Here's how the part is built. I have some questions about the finished solid (model axes, mm). Face numbers are marked on the shaded views. Round coordinates to 2 decimals unless told otherwise and drop trailing zeros. Write each loop counter-clockwise with the first axis right and the second up, starting at its lowest first coordinate (ties: lowest second). Pieces come first, ordered by that corner, then holes. Notation, with made-up numbers: (-39.5, -15) - (17.5, -15) arc R20 ccw to (17.5, 10) - close; hole circle Ø6 at (-36.75, 17.25). An arc over 180 degrees is marked (long way). Use one line per item in the form item = value. Start each with the question number.
1. I want a section at A-A, the plane x = -0.25. List the corners of the cut face in (y, z) for me.
2. I want a section at D-D, the plane z = 9. List the corners of the cut face in (x, y) for me (1 decimal), plus the area to 3 significant figures.
3. We'd pull the mould along Y, two halves only. Please class the marked faces 1, 2 and 3: +Y half, -Y half, draft (parallel to the pull), parting line (faces both ways), or undercut.
4. If I drill on line 1 along Y through (x, z) = (0, 7.75); line 2 along Y through (x, z) = (1.75, 13.25); line 3 along X through (y, z) = (8.5, 8), over which ranges is the centre line in solid material (lowest first)?
5. I want a section at B-B, the plane x = -3. List the corners of the cut face in (y, z) for me.
6. Will these pins go through, and if not, where does the flat tip stop? pin 1 (1 mm diameter, centred on x = -3, z = 20.5, fed in from -Y); pin 2 (2 mm diameter, centred on x = 4, z = 4.5, fed in from -Y); pin 3 (4 mm diameter, centred on y = 5.5, z = 3.5, fed in from -X); pin 4 (3.5 mm diameter, centred on x = 0, y = 16.59, fed in from -Z).
7. I want a section at C-C, the plane y = -1.5. List the corners of the cut face in (x, z) for me, plus the area to 3 significant figures.
```python
from build123d import *

# Parameters (mm, degrees)
SKETCH1_R           = 2.286
BOSS_EXTRUDE1_DEPTH = 25.4
SKETCH2_R           = 14.2875
CUT_EXTRUDE1_DEPTH  = 34.583444905
FILLET1_R           = 4.7625


with BuildPart() as part:
    # Sketch1 → Boss-Extrude1 (new body)
    with BuildSketch(Plane.XY):
        with BuildLine():
            Line((4.7625, 16.5862), (4.7625, 0))
            ThreePointArc((4.7625, 0), (0, -4.7625), (-4.7625, 0))
            Line((-4.7625, 0), (-4.7625, 16.5862))
            Line((-4.7625, 16.5862), (-4.7625, 21.447758984))
            Line((-4.7625, 21.447758984), (4.7625, 21.447758984))
            Line((4.7625, 21.447758984), (4.7625, 16.5862))
        make_face()
        Circle(SKETCH1_R, mode=Mode.SUBTRACT)
        with Locations((0, 16.5862)):
            Circle(SKETCH1_R, mode=Mode.SUBTRACT)
    extrude(amount=BOSS_EXTRUDE1_DEPTH)

    # Sketch2 → Cut-Extrude1 (cut, through all)
    with BuildSketch(Plane.XY.offset(25.4)):
        with Locations((-16.67002, 8.2931)):
            Circle(SKETCH2_R)
    extrude(amount=-CUT_EXTRUDE1_DEPTH, mode=Mode.SUBTRACT)

    # Fillet1
    # the kernel refuses this fillet: 4.7625 mm, written as the material it takes off along each edge
    with BuildSketch(Plane(origin=(-4.7625, 0.397302149, -2.281929285), x_dir=(0.5257327344691161, 0.8506498056824712, 0), z_dir=(0, 0, 1))) as fillet1_piece_1:
        with BuildLine():
            CenterArc((1.064900333, -4.760069656), FILLET1_R, 91.830511452, 15.300937173)
            Line((-0.337964996, -0.208874745), (-0.366022303, -0.117850847))
            ThreePointArc((-0.366022303, -0.117850847), (-0.219058541, -0.023412979), (-0.050076043, 0.081024394))
            Line((-0.050076043, 0.081024394), (0.003042572, 0.095201393))
            ThreePointArc((0.003042572, 0.095201393), (0.456385857, 0.087958969), (0.909729142, 0.095201393))
            Line((0.909729142, 0.095201393), (0.912771714, 0))
        make_face()
    extrude(amount=29.963858571, mode=Mode.SUBTRACT)
    with BuildSketch(Plane(origin=(-4.7625, 16.188897851, -3.311119953), x_dir=(0, 1, 0), z_dir=(0, 0, 1))) as fillet1_piece_2:
        with BuildLine():
            CenterArc((1.324447981, -4.7625), FILLET1_R, 90, 28.947133413)
            Line((-0.980613477, -0.594995), (-1.026714706, -0.5116449))
            ThreePointArc((-1.026714706, -0.5116449), (-0.533743292, -0.225909554), (-0.052638652, 0.079383467))
            Line((-0.052638652, 0.079383467), (0, 0.09525))
            Line((0, 0.09525), (1.324447981, 0.09525))
            Line((1.324447981, 0.09525), (1.324447981, 0))
        make_face()
    extrude(amount=32.022239906, mode=Mode.SUBTRACT)


solid = part.part
```
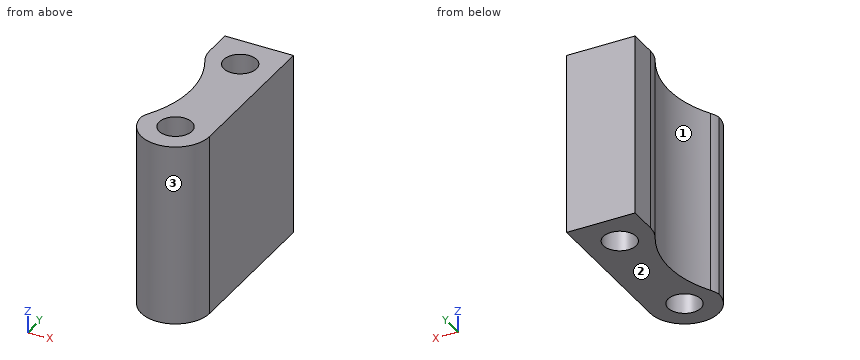
Model answer:
q1.outline = (-4.76, 0) - (-2.27, 0) - (-2.27, 25.4) - (-4.76, 25.4) - close; (2.27, 0) - (14.31, 0) - (14.31, 25.4) - (2.27, 25.4) - close; (18.86, 0) - (21.45, 0) - (21.45, 25.4) - (18.86, 25.4) - close
q2.outline = (-4.8, 0) arc R4.8 ccw to (4.8, 0) - (4.8, 21.4) - (-4.8, 21.4) - (-4.8, 17.5) arc R4.8 ccw to (-4.2, 15.2) arc R14.3 cw to (-4.3, 1.2) arc R4.8 ccw to start; hole circle Ø4.6 at (0, 0); hole circle Ø4.6 at (0, 16.6)
q2.area = 181 mm2
q3.face_1 = undercut
q3.face_2 = draft
q3.face_3 = -Y half
q4.line_1 = -4.76 to -2.29, 2.29 to 14.3, 18.87 to 21.45
q4.line_2 = -4.43 to -1.47, 1.47 to 15.12, 18.06 to 21.45
q4.line_3 = -2.38 to 4.76
q5.outline = (-3.7, 0) - (4.14, 0) - (4.14, 25.4) - (-3.7, 25.4) - close; (12.45, 0) - (21.45, 0) - (21.45, 25.4) - (12.45, 25.4) - close
q6.pin_1 = -4.05
q6.pin_2 = -3.7
q6.pin_3 = -3.21
q6.pin_4 = through
q7.outline = (-4.52, 0) - (-1.73, 0) - (-1.73, 25.4) - (-4.52, 25.4) - close; (1.73, 0) - (4.52, 0) - (4.52, 25.4) - (1.73, 25.4) - close
q7.area = 142 mm2
